The listing builds one solid part. Answer for the finished solid, in the listing's coordinates (mm). Face numbers are marked on the shaded views. A direction names the side the tool comes from. Round coordinates to 2 decimals unless told otherwise and drop trailing zeros. Order: outer loops, then holes, each group sorted by start corner. A loop starts at its lowest first (then second) coordinate and runs counter-clockwise, first axis right, second up. Notation, with made-up numbers: (76, 88) -> (133, 88) arc R23 ccw to (133, 118) -> close; hole circle Ø1 at (71, 5.5). An arc over 180 degrees is marked (long way). Return JSON: item names as keys, results as strings. Group by question number.
(1) The part is cut by section B-B (x = -34.5). Determine the outline of the cut face in (y, z).
(2) Consider line 1 (Y direction, x = 15.5, z = -9.8); line 2 (Y direction, x = -26.5, z = -9.5); line 3 (X direction, y = -6.5, z = -2). Determine where each line is inside the solid, lowest interval first. Write a range as [from, to].
(3) Determine the mould class of the marked faces 1, 2 and 3 for opening direction Y: +Y half, -Y half, draft (parallel to the pull), parting line (faces both ways), or undercut.
(4) The part is cut by section D-D (y = -16). Determine the outline of the cut face in (x, z), plus the area to 3 significant figures.
(5) Which of the six approach directions +Z, -Z, +X, -X, +Y, -Y give full straight-line access (tool end or side, diameter ignored) to the marked faces 4, 5, 6, 7 and 8?
(6) Each of these flat-tipped pins is pushed along its axis until it touches: pin 1 (3 mm diameter, centred on x = -0.5, z = -7, fed in from -Y); pin 2 (12 mm diameter, centred on x = -4, y = 4, fed in from +Z); pin 3 (4 mm diameter, centred on y = 11.5, z = -2, fed in from -X); pin 4 (3.5 mm diameter, centred on x = -34.5, y = -6, fed in from -Z). Where does it stop, or does it pass through?
(7) The part is cut by section A-A (y = 0). Determine the outline of the cut face in (x, z).
(8) The part is cut by section C-C (x = -4). Determine the outline of the cut face in (y, z).
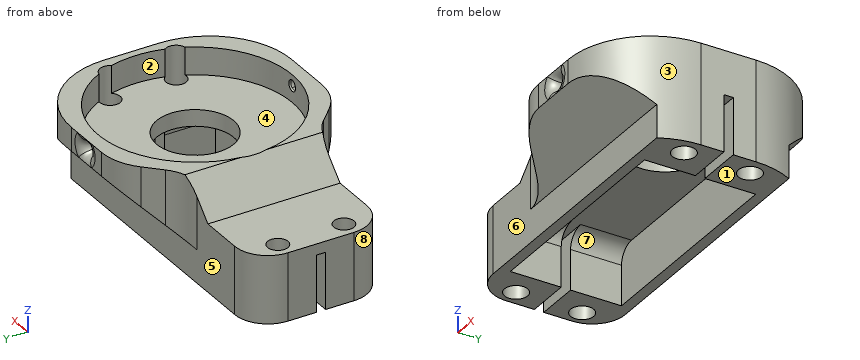
from build123d import *

# Parameters (mm, degrees)
SKETCH035_R          = 7
SKETCH035_R_2        = 1.85
PAD031_DEPTH         = 8
PAD031_DEPTH_BACK    = 10.3
POCKET036_DEPTH      = 10.1
SKETCH070_W          = 1.7
SKETCH070_H          = 20
POCKET037_DEPTH      = 56.501
SKETCH043_R          = 17.65
POCKET038_DEPTH      = 5
POCKET039_DEPTH      = 20.001
POCKET039_DEPTH_BACK = 20.001
POCKET040_DEPTH      = 167.7091
POCKET040_DEPTH_BACK = 175.2091
SKETCH073_R          = 1
POCKET041_DEPTH      = 20.001
POCKET041_DEPTH_BACK = 20.001
FILLET006_R          = 2
SKETCH074_R          = 2.1
POCKET042_DEPTH      = 3


with BuildPart() as part:
    # Sketch035 → Pad031 (new body, two sides)
    with BuildSketch(Plane.XY) as pad031_sk:
        with BuildLine():
            Line((-24.5, 6), (-24.5, -6))
            ThreePointArc((-24.5, -6), (-22.742641, -10.242641), (-18.5, -12))
            Line((-7.313708, -12), (-18.5, -12))
            ThreePointArc((-1.656854, -14.343146), (-4.252241, -12.608964), (-7.313708, -12))
            Line((-1.656854, -14.343146), (1.071068, -17.071068))
            ThreePointArc((1.071068, -17.071068), (4.315301, -19.238795), (8.142136, -20))
            Line((8.142136, -20), (17, -20))
            ThreePointArc((17, -20), (27.606602, -15.606602), (32, -5))
            Line((32, -5), (32, 5))
            ThreePointArc((32, 5), (27.606602, 15.606602), (17, 20))
            Line((8.142136, 20), (17, 20))
            ThreePointArc((8.142136, 20), (4.315301, 19.238795), (1.071068, 17.071068))
            Line((1.071068, 17.071068), (-1.656854, 14.343146))
            ThreePointArc((-7.313708, 12), (-4.252241, 12.608964), (-1.656854, 14.343146))
            Line((-7.313708, 12), (-18.5, 12))
            ThreePointArc((-18.5, 12), (-22.742641, 10.242641), (-24.5, 6))
        make_face()
        with Locations((13, 0)):
            Circle(SKETCH035_R, mode=Mode.SUBTRACT)
        with Locations((-21.5, 6)):
            Circle(SKETCH035_R_2, mode=Mode.SUBTRACT)
        with Locations((-21.5, -6)):
            Circle(SKETCH035_R_2, mode=Mode.SUBTRACT)
        with Locations((28.5, 6)):
            Circle(SKETCH035_R_2, mode=Mode.SUBTRACT)
        with Locations((28.5, -6)):
            Circle(SKETCH035_R_2, mode=Mode.SUBTRACT)
    extrude(amount=PAD031_DEPTH)
    extrude(pad031_sk.sketch, amount=-PAD031_DEPTH_BACK)

    # Sketch069 → Pocket036 (cut, symmetric)
    with BuildSketch(Plane.XZ):
        with BuildLine():
            Line((-16.5, -3), (-16.5, -20))
            Line((-16.5, -20), (23.5, -20))
            Line((23.5, -20), (23.5, -3))
            ThreePointArc((23.5, -3), (22.62132, -0.87868), (20.5, 0))
            Line((20.5, 0), (-13.5, 0))
            ThreePointArc((-13.5, 0), (-15.62132, -0.87868), (-16.5, -3))
        make_face()
    extrude(amount=POCKET036_DEPTH, both=True, mode=Mode.SUBTRACT)

    # Sketch070 (on Face7 of Pocket036) → Pocket037 (cut, through all)
    with BuildSketch(Plane(origin=(-24.5, 0, 0), x_dir=(0, -1, 0), z_dir=(-1, 0, 0))):
        with Locations((0, -10)):
            Rectangle(SKETCH070_W, SKETCH070_H)
    extrude(amount=-POCKET037_DEPTH, mode=Mode.SUBTRACT)

    # Sketch043 (on Face5 of Pocket037) → Pocket038 (cut)
    with BuildSketch(Plane.XY.offset(8)):
        with Locations((13, 0)):
            Circle(SKETCH043_R)
    extrude(amount=-POCKET038_DEPTH, mode=Mode.SUBTRACT)

    # Sketch071 → Pocket039 (cut, two sides)
    with BuildSketch(Plane.XZ) as pocket039_sk:
        Polygon((-24.5, 8), (-24.5, 2), (-10.5, 2), (-4.5, 8), align=None)
    extrude(amount=-POCKET039_DEPTH, mode=Mode.SUBTRACT)
    extrude(pocket039_sk.sketch, amount=POCKET039_DEPTH_BACK, mode=Mode.SUBTRACT)

    # Sketch072 → Pocket040 (cut, two sides)
    with BuildSketch(Plane.YZ) as pocket040_sk:
        Polygon((-20, -10.3), (-12, -10.3), (-12, -4.3), (-20, 3.7), align=None)
    pocket040 = extrude(amount=-POCKET040_DEPTH, mode=Mode.SUBTRACT) + extrude(pocket040_sk.sketch, amount=POCKET040_DEPTH_BACK, mode=Mode.SUBTRACT)

    # Mirrored005: Pocket040 across Sketch072 V_Axis
    add(pocket040.mirror(Plane(origin=(0, 0, 0), x_dir=(1, 0, 0), z_dir=(0, 1, 0))), mode=Mode.SUBTRACT)

    # Sketch073 → Pocket041 (cut, two sides)
    with BuildSketch(Plane.XZ) as pocket041_sk:
        with Locations((13, 6)):
            Circle(SKETCH073_R)
    extrude(amount=-POCKET041_DEPTH, mode=Mode.SUBTRACT)
    extrude(pocket041_sk.sketch, amount=POCKET041_DEPTH_BACK, mode=Mode.SUBTRACT)

    # Fillet006
    fillet006_edges = [part.edges().sort_by_distance(p)[0] for p in [
        (12, -20, 6),
        (12, 20, 6),
    ]]
    fillet(fillet006_edges, radius=FILLET006_R)

    # Sketch074 → Pocket042 (cut)
    with BuildSketch(Plane.XY.offset(-10.3)):
        with Locations((-21.5, 6)):
            Circle(SKETCH074_R)
        with Locations((-21.5, -6)):
            Circle(SKETCH074_R)
        with Locations((28.5, -6)):
            Circle(SKETCH074_R)
        with Locations((28.5, 6)):
            Circle(SKETCH074_R)
    extrude(amount=POCKET042_DEPTH, mode=Mode.SUBTRACT)


with BuildPart() as part_1:
    # Body018 placement: moved
    add(part.part.moved(Location((-13, 0, -0.5))))


solid = part_1.part
Answer below:
{
 "1": {"outline": "(-11.2, -10.8) -> (-8.1, -10.8) -> (-8.1, -7.8) -> (-7.85, -7.8) -> (-7.85, 1.5) -> (-11.2, 1.5) -> close; (-4.15, -7.8) -> (-3.9, -7.8) -> (-3.9, -10.8) -> (-0.85, -10.8) -> (-0.85, -0.5) -> (0.85, -0.5) -> (0.85, -10.8) -> (3.9, -10.8) -> (3.9, -7.8) -> (4.15, -7.8) -> (4.15, 1.5) -> (-4.15, 1.5) -> close; (7.85, -7.8) -> (8.1, -7.8) -> (8.1, -10.8) -> (11.2, -10.8) -> (11.2, 1.5) -> (7.85, 1.5) -> close"},
 "2": {"line 1": "y = [-12, -8.1], [-3.9, -0.85], [0.85, 3.9], [8.1, 12]", "line 2": "y = [-12, -10.1], [10.1, 12]", "line 3": "x = [-37.48, -36.28], [-32.72, -29.1], [10.1, 13.72], [17.28, 18.92]"},
 "3": {"face 1": "draft", "face 2": "undercut", "face 3": "-Y half"},
 "4": {"outline": "(-13, -0.8) -> (14.2, -0.8) -> (14.2, 7.5) -> (7.45, 7.5) -> (7.45, 2.5) -> (-7.45, 2.5) -> (-7.45, 7.5) -> (-13, 7.5) -> close", "area": "151 mm²"},
 "5": {"face 4": "+Z", "face 5": "-Z, -X, +Y", "face 6": "-Z, -X, -Y", "face 7": "-Z", "face 8": "+Z, -Z, -X, -Y"},
 "6": {"pin 1": "stops at y = -12", "pin 2": "stops at z = 2.5", "pin 3": "stops at x = -36.37", "pin 4": "passes through"},
 "7": {"outline": "(-37.5, -0.5) -> (-7, -0.5) -> (-7, 2.5) -> (-17.65, 2.5) -> (-17.65, 7.35) -> (-23.5, 1.5) -> (-37.5, 1.5) -> close; (7, -0.5) -> (19, -0.5) -> (19, 7.5) -> (17.65, 7.5) -> (17.65, 2.5) -> (7, 2.5) -> close"},
 "8": {"outline": "(-20, 3.2) -> (-12, -4.8) -> (-12, -10.8) -> (-10.1, -10.8) -> (-10.1, -0.5) -> (-5.74, -0.5) -> (-5.74, 2.5) -> (-17.19, 2.5) -> (-17.19, 7.5) -> (-20, 7.5) -> close; (5.74, -0.5) -> (10.1, -0.5) -> (10.1, -10.8) -> (12, -10.8) -> (12, -4.8) -> (20, 3.2) -> (20, 7.5) -> (17.19, 7.5) -> (17.19, 2.5) -> (5.74, 2.5) -> close"}
}
